Source: CAD feature listing. Evaluate the final solid. Frame: model axes, mm. A direction names the side the tool comes from. Give positions to 0.01 mm unless a question says otherwise; leave off trailing zeros. Answer as a JSON object with one key per item and string values. Group by question number.
from build123d import *

# Parameters (mm, degrees)
F1_DEPTH    = 76.2
F2_R        = 13.0009566934
F2_R_2      = 11.7691858669
F2_R_3      = 12.5140273394
F2_R_4      = 10.2035026267
F2_R_5      = 10.9635179416
F4_DEPTH    = 25.4
F5_T1_DEPTH = 114.7959034965
F5_T3_DEPTH = 114.5331439546
F5_T5_DEPTH = 115.5605603925
F5_T7_DEPTH = 114.7899989954


# Not quite as in the source:
# - a fillet or chamfer that OpenCascade refuses, or shapes differently, is made with other operations: its cross-section is extruded or revolved along the edge and cut away or added


with BuildPart() as f1:
    # F0 (on Front) → F1 (new body)
    with BuildSketch(Plane.XZ):
        Polygon((56.2510117888, 48.6738197505), (-33.1341587007, 49.7012361884), (-33.1341587007, -40.4544956982), (56.2510117888, -40.4544956982), align=None)
    extrude(amount=F1_DEPTH)

    # F2 (on face) → F4 (cut)
    with BuildSketch(Plane.XZ.offset(76.2)):
        with Locations((-18.2341039181, 32.6071083546)):
            Circle(F2_R)
        with Locations((36.246843636, 30.9728365391)):
            Circle(F2_R_2)
        with Locations((11.6678411141, 5.1815295592)):
            Circle(F2_R_3)
        with Locations((-18.2341039181, -19.5480342954)):
            Circle(F2_R_4)
        with Locations((33.4707759321, -15.3220649809)):
            Circle(F2_R_5)
    extrude(amount=-F4_DEPTH, mode=Mode.SUBTRACT)

    # F5: fillet of radius 5.08 on 9 edges, made by hand

    # F5_s2 → F5_t1 (cut)
    with BuildSketch(Plane(origin=(68.3857605657, 0, -0.7860437491), x_dir=(0, 1, 0), z_dir=(-0.9999339475, 0, 0.0114935013))):
        with BuildLine():
            ThreePointArc((-71.1190343146, -49.3175258025), (-74.7121024484, -47.829228251), (-76.2004, -44.2361601171))
            Line((-76.2004, -44.2361601171), (-76.7085365685, -44.2361601171))
            ThreePointArc((-76.7085365685, -44.2361601171), (-76.7081365685, -46.7766429598), (-76.7081365685, -49.3171258025))
            Line((-76.7081365685, -49.3171258025), (-76.2, -49.8252623711))
            ThreePointArc((-76.2, -49.8252623711), (-73.6595171573, -49.8252623711), (-71.1190343146, -49.8256623711))
            Line((-71.1190343146, -49.8256623711), (-71.1190343146, -49.3175258025))
        make_face()
    extrude(amount=F5_T1_DEPTH, mode=Mode.SUBTRACT)

    # F5_s4 → F5_t3 (cut)
    with BuildSketch(Plane.XY.offset(-53.1569099511)):
        with BuildLine():
            ThreePointArc((56.2514117888, -71.1190343146), (54.7631142373, -74.7121024484), (51.1700461034, -76.2004))
            Line((51.1700461034, -76.2004), (51.1700461034, -76.7085365685))
            ThreePointArc((51.1700461034, -76.7085365685), (53.7105289461, -76.7081365685), (56.2510117888, -76.7081365685))
            Line((56.2510117888, -76.7081365685), (56.7591483574, -76.2))
            ThreePointArc((56.7591483574, -76.2), (56.7591483574, -73.6595171573), (56.7595483574, -71.1190343146))
            Line((56.7595483574, -71.1190343146), (56.2514117888, -71.1190343146))
        make_face()
    extrude(amount=F5_T3_DEPTH, mode=Mode.SUBTRACT)

    # F5_s6 → F5_t5 (cut)
    with BuildSketch(Plane.XY.offset(-53.1569099511)):
        with BuildLine():
            ThreePointArc((-33.1345587007, -71.1190343146), (-31.6462611491, -74.7121024484), (-28.0531930153, -76.2004))
            Line((-28.0531930153, -76.2004), (-28.0531930153, -76.7085365685))
            ThreePointArc((-28.0531930153, -76.7085365685), (-30.593675858, -76.7081365685), (-33.1341587007, -76.7081365685))
            Line((-33.1341587007, -76.7081365685), (-33.6422952692, -76.2))
            ThreePointArc((-33.6422952692, -76.2), (-33.6422952692, -73.6595171573), (-33.6426952692, -71.1190343146))
            Line((-33.6426952692, -71.1190343146), (-33.1345587007, -71.1190343146))
        make_face()
    extrude(amount=F5_T5_DEPTH, mode=Mode.SUBTRACT)

    # F5_s8 → F5_t7 (cut)
    with BuildSketch(Plane.YZ.offset(-45.8365729536)):
        with BuildLine():
            ThreePointArc((-76.2004, -35.3735300128), (-74.7121024484, -38.9665981466), (-71.1190343146, -40.4548956982))
            Line((-71.1190343146, -40.4548956982), (-71.1190343146, -40.9630322668))
            ThreePointArc((-71.1190343146, -40.9630322668), (-73.6595171573, -40.9626322668), (-76.2, -40.9626322668))
            Line((-76.2, -40.9626322668), (-76.7081365685, -40.4544956982))
            ThreePointArc((-76.7081365685, -40.4544956982), (-76.7081365685, -37.9140128555), (-76.7085365685, -35.3735300128))
            Line((-76.7085365685, -35.3735300128), (-76.2004, -35.3735300128))
        make_face()
    extrude(amount=F5_T7_DEPTH, mode=Mode.SUBTRACT)

    # F5_s9 → F5_t10 (revolve, cut)
    with BuildSketch(Plane.XY.offset(-19.5480342954)):
        with BuildLine():
            ThreePointArc((-2.949635606, -76.2004), (-6.5427037398, -74.7121024484), (-8.0310012914, -71.1190343146))
            Line((-8.0310012914, -71.1190343146), (-8.53913786, -71.1190343146))
            ThreePointArc((-8.53913786, -71.1190343146), (-8.53873786, -73.6595171573), (-8.53873786, -76.2))
            Line((-8.53873786, -76.2), (-8.0306012914, -76.7081365685))
            ThreePointArc((-8.0306012914, -76.7081365685), (-5.4901184487, -76.7081365685), (-2.949635606, -76.7085365685))
            Line((-2.949635606, -76.7085365685), (-2.949635606, -76.2004))
        make_face()
    revolve(axis=Axis((-18.2341039181, -76.2, -19.5480342954), (0, -1, 0)), mode=Mode.SUBTRACT)

    # F5_s11 → F5_t12 (revolve, cut)
    with BuildSketch(Plane.XY.offset(-15.3220649809)):
        with BuildLine():
            ThreePointArc((49.5152595591, -76.2004), (45.9221914252, -74.7121024484), (44.4338938736, -71.1190343146))
            Line((44.4338938736, -71.1190343146), (43.9257573051, -71.1190343146))
            ThreePointArc((43.9257573051, -71.1190343146), (43.9261573051, -73.6595171573), (43.9261573051, -76.2))
            Line((43.9261573051, -76.2), (44.4342938736, -76.7081365685))
            ThreePointArc((44.4342938736, -76.7081365685), (46.9747767164, -76.7081365685), (49.5152595591, -76.7085365685))
            Line((49.5152595591, -76.7085365685), (49.5152595591, -76.2004))
        make_face()
    revolve(axis=Axis((33.4707759321, -76.2, -15.3220649809), (0, -1, 0)), mode=Mode.SUBTRACT)

    # F5_s13 → F5_t14 (revolve, cut)
    with BuildSketch(Plane.XY.offset(5.1815295592)):
        with BuildLine():
            ThreePointArc((29.2628341389, -76.2004), (25.6697660051, -74.7121024484), (24.1814684535, -71.1190343146))
            Line((24.1814684535, -71.1190343146), (23.673331885, -71.1190343146))
            ThreePointArc((23.673331885, -71.1190343146), (23.673731885, -73.6595171573), (23.673731885, -76.2))
            Line((23.673731885, -76.2), (24.1818684535, -76.7081365685))
            ThreePointArc((24.1818684535, -76.7081365685), (26.7223512962, -76.7081365685), (29.2628341389, -76.7085365685))
            Line((29.2628341389, -76.7085365685), (29.2628341389, -76.2004))
        make_face()
    revolve(axis=Axis((11.6678411141, -76.2, 5.1815295592), (0, -1, 0)), mode=Mode.SUBTRACT)

    # F5_s15 → F5_t16 (revolve, cut)
    with BuildSketch(Plane.XY.offset(32.6071083546)):
        with BuildLine():
            ThreePointArc((-0.1521815393, -76.2004), (-3.7452496731, -74.7121024484), (-5.2335472247, -71.1190343146))
            Line((-5.2335472247, -71.1190343146), (-5.7416837932, -71.1190343146))
            ThreePointArc((-5.7416837932, -71.1190343146), (-5.7412837932, -73.6595171573), (-5.7412837932, -76.2))
            Line((-5.7412837932, -76.2), (-5.2331472247, -76.7081365685))
            ThreePointArc((-5.2331472247, -76.7081365685), (-2.692664382, -76.7081365685), (-0.1521815393, -76.7085365685))
            Line((-0.1521815393, -76.7085365685), (-0.1521815393, -76.2004))
        make_face()
    revolve(axis=Axis((-18.2341039181, -76.2, 32.6071083546), (0, -1, 0)), mode=Mode.SUBTRACT)

    # F5_s17 → F5_t18 (revolve, cut)
    with BuildSketch(Plane.XY.offset(30.9728365391)):
        with BuildLine():
            ThreePointArc((53.0969951883, -76.2004), (49.5039270545, -74.7121024484), (48.0156295029, -71.1190343146))
            Line((48.0156295029, -71.1190343146), (47.5074929344, -71.1190343146))
            ThreePointArc((47.5074929344, -71.1190343146), (47.5078929344, -73.6595171573), (47.5078929344, -76.2))
            Line((47.5078929344, -76.2), (48.0160295029, -76.7081365685))
            ThreePointArc((48.0160295029, -76.7081365685), (50.5565123456, -76.7081365685), (53.0969951883, -76.7085365685))
            Line((53.0969951883, -76.7085365685), (53.0969951883, -76.2004))
        make_face()
    revolve(axis=Axis((36.246843636, -76.2, 30.9728365391), (0, -1, 0)), mode=Mode.SUBTRACT)


solid = f1.part
(1) Mould query, pull axis X, two halves, no side actions, for faces 4 (the face through (-32.24, -74, 3.99)), 5 (the face through (56.251, -35, 3)), 6 (the face through (33, -50.8, -15)), 7 (the face through (11, -35, -40.454)). Classes: pulls with the +X half, pulls with the -X half, needs draft (parallel to the pull), parting line crosses it, or undercut.
(2) First-contact query: pin 1 (3 mm diameter, centred on x = 24, y = -35.5, fed in from +Z); pin 2 (16.5 mm diameter, centred on x = -20.5, z = -17, fed in from -Y); pin 3 (2 mm diameter, centred on x = 0.5, y = -55.5, fed in from +Z). Flat tips, straight axial feed; report the tip coordinate or a pass-through.
(3) Access query for faces 1 (the face through (12.174, -74, 48.285)), 2 (the face through (26.91, -61.13, 23.81)), 3 (the face through (-33.134, -35, 5)). Directions: +Z, -Z, +X, -X, +Y, -Y. A direction counts if a zero-diameter tool reaches every point of the face in a straight line with its end or side. Return the directions, or none.
(4) Material intervals for line 1 (Z direction, x = 35.5, y = -60); line 2 (X direction, y = -52, z = -17); line 3 (Z direction, x = -19, y = -67.5), sorted ascending. Write a range as from..to.
Result:
{
 "1": {"face 4": "pulls with the -X half", "face 5": "pulls with the +X half", "face 6": "undercut", "face 7": "needs draft"},
 "2": {"pin 1": "z = 49.06", "pin 2": "y = -74.68", "pin 3": "z = 49.33"},
 "3": {"face 1": "+Z, +X, -Y", "face 2": "-Y", "face 3": "+Z, -Z, -X, +Y, -Y"},
 "4": {"line 1": "-40.45..-26.1, -4.55..19.23, 42.72..48.91", "line 2": "-33.13..-28.11, -8.35..22.64, 44.31..56.25", "line 3": "-40.45..-29.72, -9.37..19.63, 45.59..49.54"}
}
